```python
from build123d import *

# Parameters (mm, degrees)
SKETCH_1_W      = 180
SKETCH_1_H      = 180
SKETCH_1_R      = 3.4
SKETCH_1_R_2    = 8.75
EXTRUDE_1_DEPTH = 10


with BuildPart() as part:
    # 草图1 → 凸台-拉伸1 (new body)
    with BuildSketch(Plane(origin=(0, 0, 0), x_dir=(-1, 0, 0), z_dir=(0, 0, 1))):
        with Locations((65, 160)):
            Rectangle(SKETCH_1_W, SKETCH_1_H)
        with Locations(Location((145, 160, 0), (0, 0, 180))):
            Circle(SKETCH_1_R, mode=Mode.SUBTRACT)
        with Locations(Location((65, 160, 0), (0, 0, 180))):
            Circle(SKETCH_1_R, mode=Mode.SUBTRACT)
        with Locations(Location((0, 225, 0), (0, 0, 180))):
            Circle(SKETCH_1_R_2, mode=Mode.SUBTRACT)
        with Locations(Location((145, 80, 0), (0, 0, 180))):
            Circle(SKETCH_1_R, mode=Mode.SUBTRACT)
        with Locations(Location((65, 80, 0), (0, 0, 180))):
            Circle(SKETCH_1_R, mode=Mode.SUBTRACT)
    extrude(amount=EXTRUDE_1_DEPTH)


solid = part.part
```
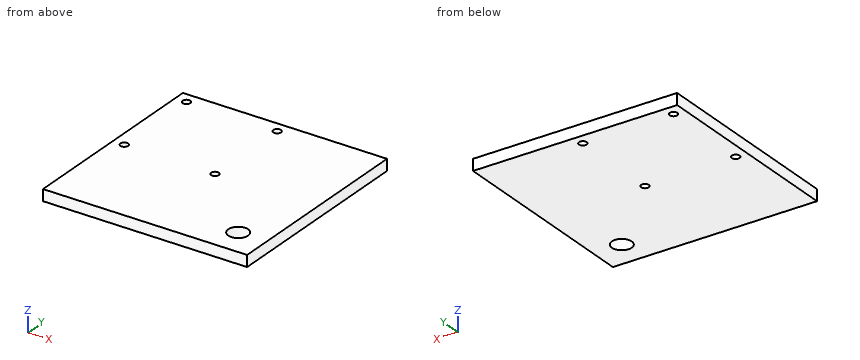
The model under review builds one solid part; all positions refer to its coordinate system, in mm. Round coordinates to 2 decimals unless told otherwise and drop trailing zeros. Write each loop counter-clockwise with the first axis right and the second up, starting at its lowest first coordinate (ties: lowest second). Pieces come first, ordered by that corner, then holes. Notation, with made-up numbers: (50.5, -10) -> (86.5, -10) arc R16 cw to (86.5, 15) -> close; hole circle Ø4 at (-6.75, 75). An arc over 180 degrees is marked (long way). Use CSV: the item, a comma, the result in double quotes.
Q1. Consider section C-C (x = 0). Give the boundary of the cut face in (y, z), then the cut area to 4 significant figures.
Checks:
outline,"(-250, 0) -> (-233.75, 0) -> (-233.75, 10) -> (-250, 10) -> close; (-216.25, 0) -> (-70, 0) -> (-70, 10) -> (-216.25, 10) -> close"
area,"1,625 mm²"
Q2. For pin 1 Ø9 at (x, y) = (-145, -80) entering from +Z, flat-tipped, find the tip position at first contact; note if it passes through.
Checks:
pin 1,"z = 10"
Q3. Consider section B-B (y = -160). Give the boundary of the cut face in (x, z).
Checks:
outline,"(-155, 0) -> (-148.4, 0) -> (-148.4, 10) -> (-155, 10) -> close; (-141.6, 0) -> (-68.4, 0) -> (-68.4, 10) -> (-141.6, 10) -> close; (-61.6, 0) -> (25, 0) -> (25, 10) -> (-61.6, 10) -> close"
Q4. To check wall thickness, follow probe 1 along Y at (x, z) = (-65, 3.5); probe 2 along Y at (x, z) = (0, 5); probe 3 along Y at (x, z) = (-3, 2.5). State the ranges of each line that lie inside material, in increasing order. Write a range as [from, to].
Checks:
probe 1,"[-250, -163.4], [-156.6, -83.4], [-76.6, -70]"
probe 2,"[-250, -233.75], [-216.25, -70]"
probe 3,"[-250, -233.22], [-216.78, -70]"
Q5. Consider section A-A (x = -65). Give the boundary of the cut face in (y, z).
Checks:
outline,"(-250, 0) -> (-163.4, 0) -> (-163.4, 10) -> (-250, 10) -> close; (-156.6, 0) -> (-83.4, 0) -> (-83.4, 10) -> (-156.6, 10) -> close; (-76.6, 0) -> (-70, 0) -> (-70, 10) -> (-76.6, 10) -> close"
